```python
from build123d import *

# Parameters (mm, degrees)
SKETCH_1_R      = 2
EXTRUDE_1_DEPTH = 10
CHAMFER_1_SIZE  = 2.5
CHAMFER_2_SIZE  = 1.5
EXTRUDE_START   = 10
EXTRUDE_2_DEPTH = 10


with BuildPart() as part:
    # 草图1 → 凸台-拉伸1 (new, symmetric)
    with BuildSketch(Plane.XY):
        with BuildLine():
            Line((-77.023496261, 32.883272305), (-77.023496261, 50))
            ThreePointArc((-77.023496261, 50), (-78.005849606, 49.902548511), (-78.949910233, 49.613992762))
            ThreePointArc((-78.949910233, 49.613992762), (-112, 0), (-78.949910233, -49.613992762))
            ThreePointArc((-78.949910233, -49.613992762), (-78.005849606, -49.902548511), (-77.023496261, -50))
            Line((-77.023496261, -50), (-77.023496261, -32.883272305))
            ThreePointArc((-77.023496261, -32.883272305), (-77.40807877, -31.413717493), (-78.463223825, -30.320939398))
            ThreePointArc((-78.463223825, -30.320939398), (-95.5, 0), (-78.463223825, 30.320939398))
            ThreePointArc((-78.463223825, 30.320939398), (-77.40807877, 31.413717493), (-77.023496261, 32.883272305))
        make_face()
        with Locations((-98.97114317, 22.5)):
            Circle(SKETCH_1_R, mode=Mode.SUBTRACT)
        with Locations((-98.97114317, -22.5)):
            Circle(SKETCH_1_R, mode=Mode.SUBTRACT)
    extrude(amount=EXTRUDE_1_DEPTH, both=True)

    # 倒角1
    chamfer_1_edges = [part.edges().sort_by_distance(p)[0] for p in [
        (-100.97114317, 22.5, 10),
        (-100.97114317, -22.5, 10),
    ]]
    chamfer(chamfer_1_edges, length=CHAMFER_1_SIZE)

    # 倒角2
    chamfer_2_edges = [part.edges().sort_by_distance(p)[0] for p in [
        (-78.005849606, 49.902548511, 10),
        (-112, 0, 10),
        (-78.005849606, -49.902548511, 10),
    ]]
    chamfer(chamfer_2_edges, length=CHAMFER_2_SIZE)

    # 草图4 → 凸台-拉伸2 (add)
    with BuildSketch(Plane.XY.offset(EXTRUDE_START)):
        with BuildLine():
            Line((-78.463223825, -30.320939398), (-78.463223825, 30.320939398))
            ThreePointArc((-78.463223825, 30.320939398), (-95.5, 0), (-78.463223825, -30.320939398))
        make_face()
    extrude(amount=-EXTRUDE_2_DEPTH)


solid = part.part
```
Geometry: final body of the model. Coordinates: model frame, mm. A direction names the side the tool comes from. Round coordinates to 2 decimals unless told otherwise and drop trailing zeros. Write each loop counter-clockwise with the first axis right and the second up, starting at its lowest first coordinate (ties: lowest second). Pieces come first, ordered by that corner, then holes.
Item 1: Section query A-A (z = -3). Return loops of the section in (x, y), plus the area to 3 significant figures.
Item 2: Section query C-C (z = 6.5). Return loops of the section in (x, y).
Item 3: Pin query (flat end, axial travel): P1, Ø10, axis at x = -91, z = 7.5, coming from the +Y side; P2, Ø3, axis at x = -90.5, z = -3, coming from the -Y side; P3, Ø8.5, axis at x = -86, y = 11, coming from the -Z side; P4, Ø3.5, axis at x = -98.97, y = 22.5, coming from the -Z side. Return the tip coordinate at first contact, or that it passes through.
Item 4: Mould query, pull axis X, two halves, no side actions, for faces 1 (the face through (-100.4, 23.9, -1.4)), 2 (the face through (-90, 1, 10)), 3 (the face through (-77.4, -31.43, 0.14)). Classes: +X half, -X half, draft (parallel to the pull), parting line (faces both ways), or undercut.
Item 5: Section query B-B (x = -98). Give the number of separate pieces and of enclosed holes in the cut face, plus the area to 3 significant figures.
Item 6: Material intervals for L1, parallel to Y at x = -98, z = -1.5; L2, parallel to Z at x = -81.5, y = 7; L3, parallel to Y at x = -80.5, z = -6.5, sorted ascending.
Item 7: Set-up query: faces 4 (the face through (-95.496, -0.509, -4.93)), 5 (the face through (-99, 1, -10)), 6 (the face through (-77.419, 31.395, 0.14)). Return all of +Z, -Z, +X, -X, +Y, -Y with unobstructed straight access to the full face (end or side cutting, diameter ignored); none if empty.
Completed:
1. outline: (-78.95, -49.61) arc R5 ccw to (-77.02, -50) - (-77.02, -32.88) arc R3 ccw to (-78.46, -30.32) arc R35.5 cw to (-78.46, 30.32) arc R3 ccw to (-77.02, 32.88) - (-77.02, 50) arc R5 ccw to (-78.95, 49.61) arc R53.76 ccw to start; hole circle Ø4 at (-98.97, -22.5); hole circle Ø4 at (-98.97, 22.5)
1. area: 1,720 mm2
2. outline: (-78.95, -49.61) arc R5 ccw to (-77.02, -50) - (-77.02, -32.88) arc R3 ccw to (-78.46, -30.32) - (-78.46, 30.32) arc R3 ccw to (-77.02, 32.88) - (-77.02, 50) arc R5 ccw to (-78.95, 49.61) arc R53.76 ccw to start; hole circle Ø4 at (-98.97, -22.5); hole circle Ø4 at (-98.97, 22.5)
3. P1: stops at y = 46.04
3. P2: stops at y = -44.09
3. P3: stops at z = 0
3. P4: passes through
4. face 1: undercut
4. face 2: draft
4. face 3: +X half
5. separate pieces: 3
5. enclosed holes: 0
5. area: 1,290 mm2
6. L1: y = -36.19 to -24.25, -20.75 to 20.75, 24.25 to 36.19
6. L2: z = 0 to 10
6. L3: y = -48.94 to -28.98, 28.98 to 48.94
7. face 4: -Z, +X
7. face 5: -Z, +X, -X, +Y, -Y
7. face 6: +Z, -Z, +X
